Work out the finished part from the listing and answer in its coordinate system (mm). Coordinates: 2 decimals unless noted, no trailing zeros. Loops run counter-clockwise (first coordinate to the right, second up) from the corner with the lowest first, then second, coordinate; pieces in that order, holes last. Notation, with made-up numbers: (-30, 6) - (-5, 6) arc R8 ccw to (-5, 21) - close; hole circle Ø11 at (48, -15). An arc over 180 degrees is marked (long way). Write each question's results on one line, items separated by ' | '. Start each with the question number.
Item 1: Section D-D, the plane x = -2.25 is taken. Write down the section's boundary in (y, z), plus the area to 3 significant figures.
Item 2: Section C-C, the plane z = -0.4 is taken. Write down the section's boundary in (x, y).
Item 3: Each of these flat-tipped pins is pushed along its axis until it touches: pin 1 Ø1.2 at (x, z) = (0.5, 1.5) entering from +Y; pin 2 Ø0.8 at (y, z) = (1, 1.5) entering from +X; pin 3 Ø3 at (x, y) = (2.5, 7) entering from +Z. Where does it stop, or does it pass through?
Item 4: Section A-A, the plane y = 8 is taken. Write down the section's boundary in (x, z).
Item 5: Consider probe 1 along Y at (x, z) = (8, -0.05); probe 2 along Y at (x, z) = (-7.5, 0.25); probe 3 along X at (y, z) = (-1.25, 1.95). Determine where each line is inside the solid, lowest interval first. Write a range as [from, to].
from build123d import *

# Parameters (mm, degrees)
SKETCH_1_W      = 23
SKETCH_1_H      = 23
SKETCH_1_R      = 1.25
EXTRUDE_1_DEPTH = 0.75
SKETCH_2_W      = 6
SKETCH_2_H      = 5
EXTRUDE_2_DEPTH = 1.5


with BuildPart() as part:
    # 草图1 → 凸台-拉伸1 (new, symmetric)
    with BuildSketch(Plane.XY):
        Rectangle(SKETCH_1_W, SKETCH_1_H)
        with Locations((-8, 8)):
            Circle(SKETCH_1_R, mode=Mode.SUBTRACT)
        with Locations((8, 8)):
            Circle(SKETCH_1_R, mode=Mode.SUBTRACT)
        with Locations((8, -8)):
            Circle(SKETCH_1_R, mode=Mode.SUBTRACT)
        with Locations((-8, -8)):
            Circle(SKETCH_1_R, mode=Mode.SUBTRACT)
    extrude(amount=EXTRUDE_1_DEPTH, both=True)

    # 草图2 → 凸台-拉伸2 (add)
    with BuildSketch(Plane.XY.offset(0.75)):
        Rectangle(SKETCH_2_W, SKETCH_2_H)
    extrude(amount=EXTRUDE_2_DEPTH)


solid = part.part
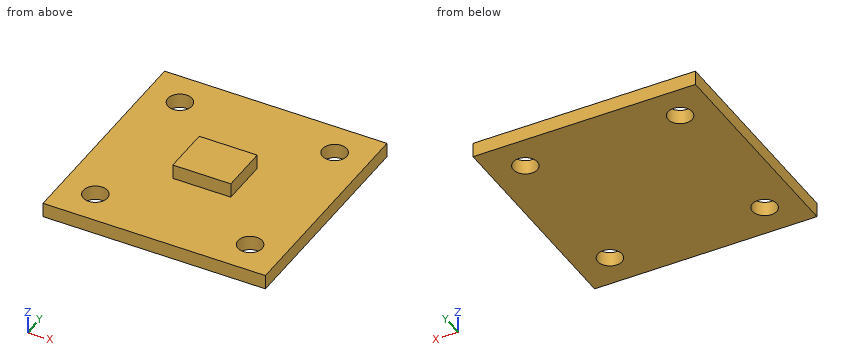
Answer key:
1) outline: (-11.5, -0.75) - (11.5, -0.75) - (11.5, 0.75) - (2.5, 0.75) - (2.5, 2.25) - (-2.5, 2.25) - (-2.5, 0.75) - (-11.5, 0.75) - close | area: 42.0 mm^2
2) outline: (-11.5, -11.5) - (11.5, -11.5) - (11.5, 11.5) - (-11.5, 11.5) - close; hole circle Ø2.5 at (-8, -8); hole circle Ø2.5 at (-8, 8); hole circle Ø2.5 at (8, -8); hole circle Ø2.5 at (8, 8)
3) pin 1: stops at y = 2.5 | pin 2: stops at x = 3 | pin 3: stops at z = 0.75
4) outline: (-11.5, -0.75) - (-9.25, -0.75) - (-9.25, 0.75) - (-11.5, 0.75) - close; (-6.75, -0.75) - (6.75, -0.75) - (6.75, 0.75) - (-6.75, 0.75) - close; (9.25, -0.75) - (11.5, -0.75) - (11.5, 0.75) - (9.25, 0.75) - close
5) probe 1: y = [-11.5, -9.25], [-6.75, 6.75], [9.25, 11.5] | probe 2: y = [-11.5, -9.15], [-6.85, 6.85], [9.15, 11.5] | probe 3: x = [-3, 3]
